from build123d import *

# Parameters (mm, degrees)
BOSS_EXTRUDE1_DEPTH = 6.35


with BuildPart() as part:
    # Elevator Belt Backplate → Boss-Extrude1 (new body)
    with BuildSketch(Plane(origin=(0, 0, 0), x_dir=(1, 0, 0), z_dir=(0, 1, 0))):
        Polygon((-31.75, -120.65), (31.75, -120.65), (31.75, -80.518), (38.1, -80.518), (38.1, -74.168), (31.75, -74.168), (31.75, -67.818), (26.215000021, -67.818), (26.215000021, -69.858999982), (23.314999979, -69.858999982), (23.314999979, -67.818), (17.78, -67.818), (17.78, -63.5), (23.314999979, -63.5), (23.314999979, -61.459000018), (26.215000021, -61.459000018), (26.215000021, -63.5), (31.75, -63.5), (31.75, 63.5), (26.215000021, 63.5), (26.215000021, 61.459000018), (23.314999979, 61.459000018), (23.314999979, 63.5), (17.78, 63.5), (17.78, 67.818), (23.314999979, 67.818), (23.314999979, 69.858999982), (26.215000021, 69.858999982), (26.215000021, 67.818), (31.75, 67.818), (31.75, 74.168), (38.1, 74.168), (38.1, 80.518), (31.75, 80.518), (31.75, 120.65), (-31.75, 120.65), (-31.75, 80.518), (-38.1, 80.518), (-38.1, 74.168), (-31.75, 74.168), (-31.75, 67.818), (-26.215000021, 67.818), (-26.215000021, 69.858999982), (-23.314999979, 69.858999982), (-23.314999979, 67.818), (-17.78, 67.818), (-17.78, 63.5), (-23.314999979, 63.5), (-23.314999979, 61.459000018), (-26.215000021, 61.459000018), (-26.215000021, 63.5), (-31.75, 63.5), (-31.75, -63.5), (-26.215000021, -63.5), (-26.215000021, -61.459000018), (-23.314999979, -61.459000018), (-23.314999979, -63.5), (-17.78, -63.5), (-17.78, -67.818), (-23.314999979, -67.818), (-23.314999979, -69.858999982), (-26.215000021, -69.858999982), (-26.215000021, -67.818), (-31.75, -67.818), (-31.75, -74.168), (-38.1, -74.168), (-38.1, -80.518), (-31.75, -80.518), align=None)
    extrude(amount=BOSS_EXTRUDE1_DEPTH)


solid = part.part
Input: part model. Units: mm. Frame: model coordinates. A direction names the side the tool comes from. Round coordinates to 2 decimals unless told otherwise and drop trailing zeros. Order: outer loops, then holes, each group sorted by start corner. A loop starts at its lowest first (then second) coordinate and runs counter-clockwise, first axis right, second up. Notation, with made-up numbers: (58, 61) - (89, 61) arc R29 ccw to (89, 100) - close; hole circle Ø7 at (64.5, -37.75). An arc over 180 degrees is marked (long way). Answer as a JSON object with one key per item and string values. Group by question number.
(1) Pin query (flat end, axial travel): P1, Ø1.9, axis at y = 3, z = -92.5, coming from the -X side; P2, Ø1.6, axis at y = 2, z = 69, coming from the +X side; P3, Ø3, axis at x = 33.5, y = 2.5, coming from the +Z side. Return the tip coordinate at first contact, or that it passes through.
(2) Cut plane A-A (z = 15.5). Return loops of the section in (x, y), then the cut area to 3 significant figures.
(3) Draft query along Z for faces 4 (the face through (35, 3, 74.168)), 5 (the face through (35, 3, -80.518)), 6 (the face through (0, 3, 120.65)). Return one class per face: released by +Z, released by -Z, zero draft, split by the parting line, or undercut.
(4) Material intervals for probe 1 along Z at (x, y) = (20, 4); probe 2 along Z at (x, y) = (25.5, 0.75); probe 3 along X at (y, z) = (4.75, 69.5) (3 decimals), sorted ascending. Write a range as from..to.
(5) Reachability of faces 1 (the face through (38.1, 3, 77)), 2 (the face through (31.75, 3, -71)), 3 (the face through (-35, 3, 74.168)) from +Z, -Z, +X, -X, +Y, -Y: full face, straight path, thin tool, end or side. Return the list, or none.
Here are the results:
{
 "1": {"P1": "stops at x = -31.75", "P2": "stops at x = 31.75", "P3": "stops at z = 80.52"},
 "2": {"outline": "(-31.75, 0) - (31.75, 0) - (31.75, 6.35) - (-31.75, 6.35) - close", "area": "403 mm^2"},
 "3": {"face 4": "undercut", "face 5": "released by -Z", "face 6": "released by +Z"},
 "4": {"probe 1": "z = -120.65..-67.82, -63.5..63.5, 67.82..120.65", "probe 2": "z = -120.65..-69.86, -61.46..61.46, 69.86..120.65", "probe 3": "x = -31.75..-26.215, -23.315..23.315, 26.215..31.75"},
 "5": {"face 1": "+Z, -Z, +X, +Y, -Y", "face 2": "+X, +Y, -Y", "face 3": "-X, +Y, -Y"}
}
